Autodesk Fusion 360 part; units mm, degrees
sketch "Sketch1" plane through (0, 0, 0) normal (1, 0, 0) x (0, 1, 0)
  circle A0 centre (0, 0) radius 80
  dimension "d1" = 160
extrude "Extrude1" add sketch "Sketch1" along normal blind 3 makes body 1
copy_body "Body->Comp1" bodies 1 removing the originals makes body 2 in component "Component"
sketch "Sketch2" plane through (3, 0, 0) normal (1, 0, 0) x (0, 1, 0)
  circle A0 centre (0, 0) radius 80
  circle A1 centre (0, 0) radius 3
  dimension "d4" = 6
extrude "Extrude1'" cut sketch "Sketch2" against normal blind 10 contours A1 bodies 2 in component "Component"
sketch "Sketch3" plane through (3, 0, 0) normal (1, 0, 0) x (0, 1, 0)
  circle A0 centre (0, 0) radius 3
  circle A1 centre (0, 0) radius 80
  circle A2 centre (0, 0) radius 75
  circle A3 centre (0, 0) radius 8
  line L0 (-5, 77.486) -> (5, 77.486)
  line L1 (5, 77.486) -> (5, -77.486)
  line L2 (5, -77.486) -> (-5, -77.486)
  line L3 (-5, -77.486) -> (-5, 77.486)
  line L4 (-5, 77.486) -> (5, -77.486) construction
  line L5 (5, 77.486) -> (-5, -77.486) construction
  line L6 (-77.0993, 5) -> (77.0993, 5)
  line L7 (77.0993, 5) -> (77.0993, -5)
  line L8 (77.0993, -5) -> (-77.0993, -5)
  line L9 (-77.0993, -5) -> (-77.0993, 5)
  line L10 (-77.0993, 5) -> (77.0993, -5) construction
  line L11 (77.0993, 5) -> (-77.0993, -5) construction
  dimension "d7" = 150
  dimension "d8" = 16
  dimension "d9" = 10
  dimension "d10" = 10
extrude "Extrude2" cut sketch "Sketch3" against normal blind 40 contours A2 A3 L1 L6 | A2 A3 L1 L8 bodies 2 in component "Component"
extrude "Extrude3" add 1 faces at (3, -2.6006, 53.0241) along direction (1, 0, 0) blind 5 on bodies 2 bodies 2 in component "Component"
component "Component" placed x (1, 0, 0) y (0, 1, 0) z (0, 0, 1) at (0, 0, 0)
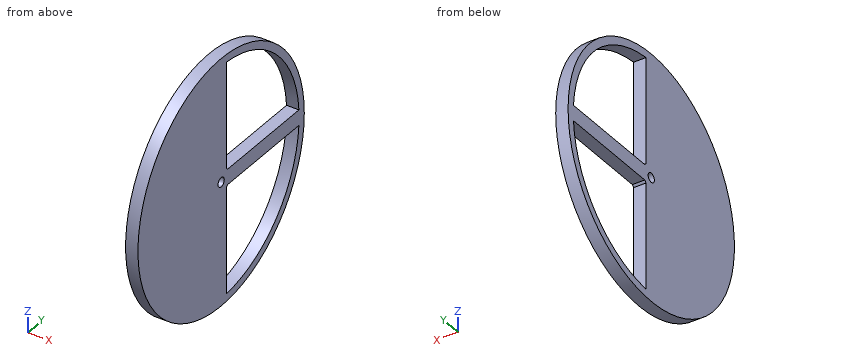
Could you check a few things on this model? Use its own coordinates, in mm. Round coordinates to 2 decimals unless told otherwise and drop trailing zeros. Write each loop counter-clockwise with the first axis right and the second up, starting at its lowest first coordinate (ties: lowest second). Pieces come first, ordered by that corner, then holes. Notation, with made-up numbers: M -27.75,13.5 L -5.75,13.5 A17 ccw -5.75,40.5 Z; hole C 87.25,4 d1. An arc over 180 degrees is marked long. Answer in a Markdown table with one row per item. Add a question column.
Q1. Imagine slicing it at A-A (z = 18). Please give me the cut outline in (x, y).
Q2. If I drill on line 1 (Z direction, x = 3, y = 0); line 2 (Z direction, x = 4.25, y = 50.5); line 3 (Z direction, x = 5, y = -1), over which ranges is the centre line in solid material (lowest first)? Write a range as from..to.
Q3. Will these pins go through, and if not, where does the flat tip stop? pin 1 Ø2 at (x, y) = (2.5, -22.5) entering from +Z; pin 2 Ø1.5 at (x, y) = (3.5, -2) entering from -Z; pin 3 Ø1.5 at (x, z) = (3.5, 35.5) entering from -Y.
Q4. Imagine slicing it at B-B (y = 0). Please give me the cut outline in (x, z), then the cut area to 3 significant figures.
Q5. Imagine slicing it at C-C (x = 3.5). Please give me the cut outline in (y, z) (3 decimals).
Q6. Imagine slicing it at D-D (y = 37). Please give me the cut outline in (x, z).
Values:
| question | item | result |
|---|---|---|
| 1 | outline | M 0,-77.95 L 8,-77.95 L 8,5 L 0,5 Z; M 0,72.81 L 8,72.81 L 8,77.95 L 0,77.95 Z |
| 2 | line 1 | -80..-3, 3..80 |
| 2 | line 2 | -62.05..-55.45, -5..5, 55.45..62.05 |
| 2 | line 3 | -79.99..-2.83, 2.83..79.99 |
| 3 | pin 1 | z = 77.06 |
| 3 | pin 2 | z = -79.99 |
| 3 | pin 3 | y = -72.06 |
| 4 | outline | M 0,-80 L 8,-80 L 8,-3 L 0,-3 Z; M 0,3 L 8,3 L 8,80 L 0,80 Z |
| 4 | area | 1,230 mm^2 |
| 5 | outline | C 0,0 d160; hole C 0,0 d6; hole M 5,-74.833 A75 ccw 74.833,-5 L 6.245,-5 A8 cw 5,-6.245 Z; hole M 5,6.245 A8 cw 6.245,5 L 74.833,5 A75 ccw 5,74.833 Z |
| 6 | outline | M 0,-70.93 L 8,-70.93 L 8,-65.24 L 0,-65.24 Z; M 0,-5 L 8,-5 L 8,5 L 0,5 Z; M 0,65.24 L 8,65.24 L 8,70.93 L 0,70.93 Z |
